Source: CAD feature listing. Evaluate the final solid. Frame: model axes, mm. Coordinates: 2 decimals unless noted, no trailing zeros. Loops run counter-clockwise (first coordinate to the right, second up) from the corner with the lowest first, then second, coordinate; pieces in that order, holes last.
Item 1: Pin query (flat end, axial travel): pin 1 Ø11 at (x, z) = (0, 61.5) entering from +Y; pin 2 Ø5 at (x, z) = (0.5, -63) entering from +Y; pin 3 Ø1.1 at (x, y) = (-27, -0.5) entering from -Z; pin 4 Ø2.5 at (x, z) = (158.5, 1.5) entering from -Y. Return the tip coordinate at first contact, or that it passes through.
Item 2: Line query: probe 1 along Y at (x, z) = (101.5, -29.5); probe 2 along X at (y, z) = (12, 0); probe 3 along X at (y, z) = (3.75, -3.5). Output: solid intervals per line, ascending.
Item 3: Section query B-B, the plane z = 39. Return the cut outline in (x, y), then the cut area to 3 significant figures.
Item 4: Section query A-A, the plane y = 21.75. Return the cut outline in (x, z), then the cut area to 3 significant figures.
Item 5: Section query C-C, the plane x = 50. Return the cut outline in (y, z), then the cut area to 3 significant figures.
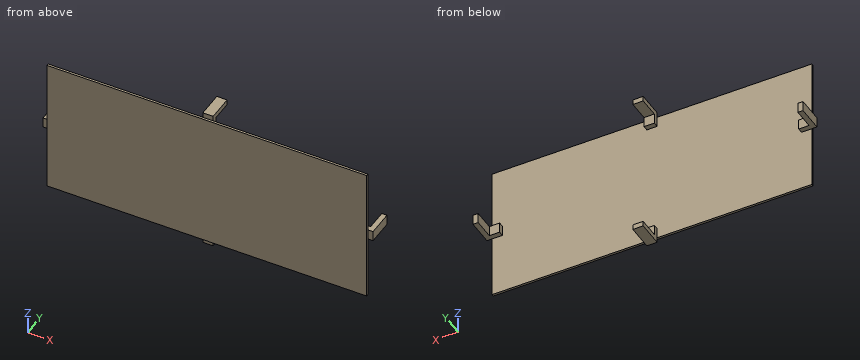
```python
from build123d import *

# Parameters (mm, degrees)
F0_W     = 310
F0_H     = 133
F1_DEPTH = 1.07
F2_W     = 10
F2_H     = 15
F2_W_2   = 15
F2_H_2   = 10
F3_DEPTH = 5
F4_W     = 5
F4_H     = 10
F4_W_2   = 10
F4_H_2   = 5
F5_DEPTH = 20


with BuildPart() as f1:
    # F0 (on Front) → F1 (new body, symmetric)
    with BuildSketch(Plane.XZ):
        Rectangle(F0_W, F0_H)
    extrude(amount=F1_DEPTH, both=True)

    # F2 (on face) → F3 (join)
    with BuildSketch(Plane(origin=(0, 1.07, 0), x_dir=(-1, 0, 0), z_dir=(0, 1, 0))):
        with Locations((0, 64)):
            Rectangle(F2_W, F2_H)
        with Locations((-152.5, 0)):
            Rectangle(F2_W_2, F2_H_2)
        with Locations((0, -64)):
            Rectangle(F2_W, F2_H)
        with Locations((152.5, 0)):
            Rectangle(F2_W_2, F2_H_2)
    extrude(amount=F3_DEPTH)

    # F4 (on face) → F5 (join)
    with BuildSketch(Plane(origin=(0, 6.07, 0), x_dir=(-1, 0, 0), z_dir=(0, 1, 0))):
        with Locations((-157.5, 0)):
            Rectangle(F4_W, F4_H)
        with Locations((157.5, 0)):
            Rectangle(F4_W, F4_H)
        with Locations((0, 69)):
            Rectangle(F4_W_2, F4_H_2)
        with Locations((0, -69)):
            Rectangle(F4_W_2, F4_H_2)
    extrude(amount=F5_DEPTH)


solid = f1.part
```
Verdict:
1. pin 1: stops at y = 26.07
1. pin 2: stops at y = 6.07
1. pin 3: stops at z = -66.5
1. pin 4: stops at y = 1.07
2. probe 1: y = -1.07 to 1.07
2. probe 2: x = -160 to -155, 155 to 160
2. probe 3: x = -160 to -145, 145 to 160
3. outline: (-155, -1.07) - (155, -1.07) - (155, 1.07) - (-155, 1.07) - close
3. area: 663 mm2
4. outline: (-160, -5) - (-155, -5) - (-155, 5) - (-160, 5) - close; (-5, -71.5) - (5, -71.5) - (5, -66.5) - (-5, -66.5) - close; (-5, 66.5) - (5, 66.5) - (5, 71.5) - (-5, 71.5) - close; (155, -5) - (160, -5) - (160, 5) - (155, 5) - close
4. area: 200 mm2
5. outline: (-1.07, -66.5) - (1.07, -66.5) - (1.07, 66.5) - (-1.07, 66.5) - close
5. area: 285 mm2
